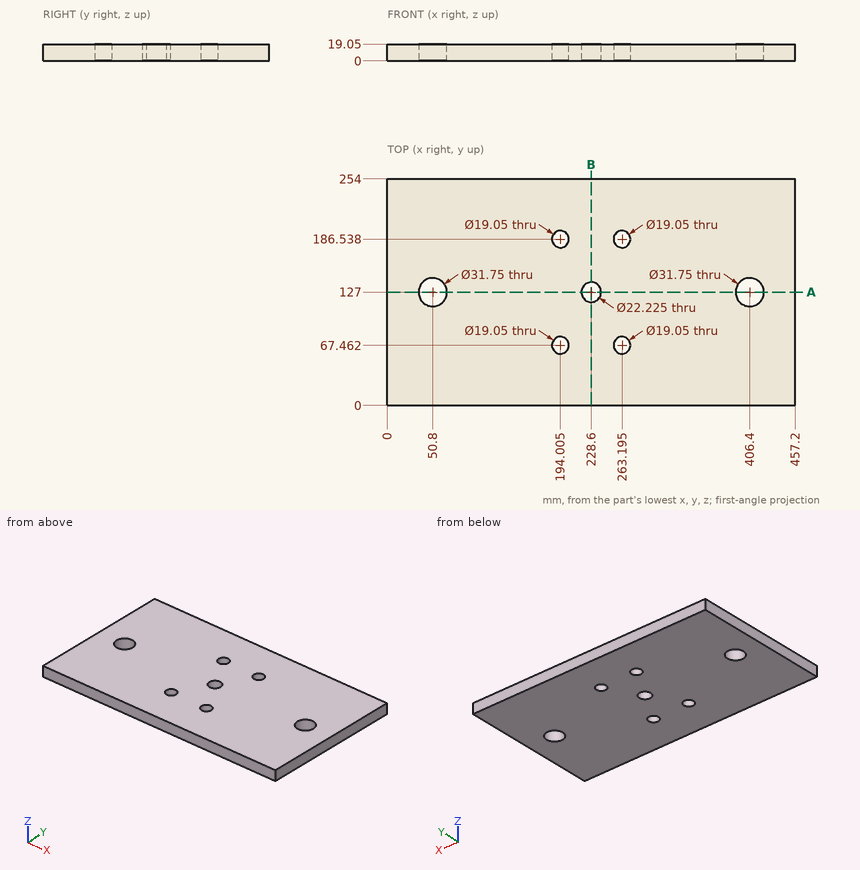
Verification items for this drawing (mm, ordinates from the low corner). Give positions to 0.01 mm unless a question says otherwise; leave off trailing zeros. Loops run counter-clockwise (first coordinate to the right, second up) from the corner with the lowest first, then second, coordinate; pieces in that order, holes last. Notation, with made-up numbers: M 26.25,45.25 L 61.25,45.25 A15 ccw 61.25,68.25 Z; hole C -39,29 d2. An arc over 180 degrees is marked long. Write item = value, one per line.
(1) Sectioned sample at A-A, the plane y = 127. State how many separate pieces and enclosed holes the cut face has, plus the area to 3 significant figures.
Answer below:
separate_pieces = 4
enclosed_holes = 0
area = 7,080 mm2
(2) Material ranges on line 1 (X direction, y = 114.5, z = 2.5) (1 decimal); line 2 (Y direction, x = 261.5, z = 17) (1 decimal); line 3 (Y direction, x = 228.6, z = 7.25), recorded low to high. Write a range as [from, to].
Answer below:
line_1 = [0, 41], [60.6, 396.6], [416.2, 457.2]
line_2 = [0, 58.1], [76.8, 177.2], [195.9, 254]
line_3 = [0, 115.89], [138.11, 254]
(3) Sectioned sample at B-B, the plane x = 228.6. Record the cut outline in (y, z).
Answer below:
outline = M 0,0 L 115.89,0 L 115.89,19.05 L 0,19.05 Z; M 138.11,0 L 254,0 L 254,19.05 L 138.11,19.05 Z
(4) Gauge pin test, flat end, axial feed: pin 1 Ø19 at (x, y) = (50.8, 127) entering from -Z. Record the tip position at first contact, or that the pin passes through.
Answer below:
pin_1 = through
